Autodesk Inventor part; units mm, degrees
ref_plane "YZ Plane" through (0, 0, 0) normal (1, 0, 0) x (0, 1, 0)
ref_plane "XZ Plane" through (0, 0, 0) normal (0, 1, 0) x (-1, 0, 0)
ref_plane "XY Plane" through (0, 0, 0) normal (0, 0, 1) x (1, 0, 0)
sketch "Sketch1" plane through (0, 0, 0) normal (0, 0, 1) x (1, 0, 0)
  line L0 (3.25, -3.75) -> (-3.25, -3.75)
  line L1 (-3.75, -3.25) -> (-3.75, 3.25)
  line L2 (-3.25, 3.75) -> (3.25, 3.75)
  line L3 (3.75, 3.25) -> (3.75, -3.25)
  line L4 (3.75, -3.75) -> (-3.75, 3.75) construction
  line L5 (-3.75, -3.75) -> (3.75, 3.75) construction
  arc A0 (-3.25, 3.75) -> (-3.75, 3.25) centre (-3.25, 3.25) ccw
  arc A1 (-3.75, -3.25) -> (-3.25, -3.75) centre (-3.25, -3.25) ccw
  arc A2 (3.25, -3.75) -> (3.75, -3.25) centre (3.25, -3.25) ccw
  arc A3 (3.75, 3.25) -> (3.25, 3.75) centre (3.25, 3.25) ccw
  point P0 (0, 0)
  dimension "d0" = 7.5
  dimension "d1" = 0.5
extrude "Extrusion1" add sketch "Sketch1" along normal mid plane 3.02
sketch "Sketch2" plane through (0, 0, -1.51) normal (0, 0, -1) x (-1, 0, 0)
  line L0 (2.96, -3) -> (1.56, -3)
  line L1 (1.56, -3) -> (1.56, 3)
  line L2 (1.56, 3) -> (2.96, 3)
  line L3 (2.96, 3) -> (2.96, -3)
  line L4 (-1.56, -3) -> (-2.96, -3)
  line L5 (-2.96, -3) -> (-2.96, 3)
  line L6 (-2.96, 3) -> (-1.56, 3)
  line L7 (-1.56, 3) -> (-1.56, -3)
  line L8 (0, -3) -> (0, 3) construction
  point P0 (0, 0)
  point P1 (0, 0)
  dimension "d4" = 1.4
  dimension "d5" = 6
  dimension "d6" = 3.12
extrude "Extrusion2" add sketch "Sketch2" along normal blind 0.08
sketch "Sketch3" plane through (0, 0, 1.51) normal (0, 0, 1) x (1, 0, 0)
  line L0 (2.75, 2.5) -> (2.5, 2.5)
  line L1 (2.5, 2.5) -> (2.5, -2.5)
  line L2 (2.5, -2.5) -> (2.75, -2.5)
  line L3 (2.75, -2.5) -> (2.75, 2.5)
  line L4 (-2.5, 2.5) -> (-2.5, -2.5) construction
  spline S0 degree 4 poles (1.3361, 0.4296) (1.5722, 0.2536) (1.6111, 0.0081) (1.8752, -0.3041) (1.3349, -0.7643) (0.9016, -0.6061) (0.6086, -0.3512) (0.6279, 0.0301) (0.8528, 0.1857) (1.2221, 0.0137) (1.0663, -0.2096) (0.9971, -0.1716) (0.8339, -0.0827) (0.9372, -0.3475) (1.124, -0.4244) (1.5104, -0.4795) (1.4218, 0.1865) (0.9203, 0.4463) (0.2397, 0.5724) (-0.0703, -0.2361) (0.2655, -0.4716) (0.366, -0.6909) (0.4591, -0.7727) knots 0 0 0 0 0 0.123761 0.174234 0.226685 0.279962 0.33014 0.377129 0.419078 0.455262 0.487036 0.514913 0.545248 0.580512 0.622872 0.674906 0.733244 0.796807 0.860625 0.919671 1 1 1 1 1
  line L5 (0.3021, -0.6347) -> (0.6161, -0.9108) construction
  arc A0 (0.3672, -0.6474) -> (0.5952, -0.8479) centre (0.698, -0.5011) ccw construction
  spline S1 degree 4 poles (1.3361, 0.4296) (1.1748, 0.5523) (0.7861, 0.8379) (-0.1178, 0.7487) (-0.2762, -0.1647) (0.0057, -0.6403) (0.1538, -0.7727) knots 0 0 0 0 0 0.46045 0.670358 1 1 1 1 1
  line L6 (-0.0024, -0.6331) -> (0.3101, -0.9124) construction
  arc A1 (0.0518, -0.6477) -> (0.2895, -0.8602) centre (0.4983, -0.3874) ccw construction
  line L7 (0.4591, -0.7727) -> (0.1538, -0.7727)
  line L8 (1.4819, -0.2272) -> (1.2942, 0.2269) construction
  arc A2 (1.4343, -0.1846) -> (1.2905, 0.1631) centre (0.7871, -0.2485) ccw construction
  line L9 (-2.1499, 0.6983) -> (-2.1499, 0.9013)
  line L10 (-2.1499, 0.9013) -> (-2.5036, 0.9013)
  line L11 (-2.5036, 0.9013) -> (-2.5036, 1.2648)
  line L12 (-2.5036, 1.2648) -> (-2.1499, 1.2648)
  line L13 (-2.1499, 1.2648) -> (-2.1499, 1.9261)
  line L14 (-2.1499, 1.9261) -> (-1.8703, 1.9261)
  line L15 (-1.8703, 1.9261) -> (-1, 1.2769)
  line L16 (-1, 1.2769) -> (-1, 0.9013)
  line L17 (-1, 0.9013) -> (-1.8801, 0.9013)
  line L18 (-1.8801, 0.9013) -> (-1.8801, 0.6983)
  line L19 (-1.8801, 0.6983) -> (-2.1499, 0.6983)
  line L20 (-1.8801, 1.2648) -> (-1.3695, 1.2648)
  line L21 (-1.3695, 1.2648) -> (-1.8801, 1.6453)
  line L22 (-1.8801, 1.6453) -> (-1.8801, 1.2648)
  line L23 (-1.2978, -0.5646) -> (-2.5, 0.076)
  line L24 (-2.5, 0.076) -> (-2.5, 0.4941)
  line L25 (-2.5, 0.4941) -> (-1.2832, -0.1756)
  line L26 (-1.2832, -0.1756) -> (-1.2832, 0.5391)
  line L27 (-1.2832, 0.5391) -> (-1, 0.5391)
  line L28 (-1, 0.5391) -> (-1, -0.5646)
  line L29 (-1, -0.5646) -> (-1.2978, -0.5646)
  line L30 (-2.5, -1.9115) -> (-2.5, -0.809)
  line L31 (-2.5, -0.809) -> (-2.2557, -0.809)
  spline S2 degree 2 poles (-2.2557, -0.809) (-2.1438, -0.9487) (-1.9469, -1.1724) (-1.8582, -1.2563) knots 0 0 0 1 2 2 2
  spline S3 degree 2 poles (-1.8582, -1.2563) (-1.7427, -1.3669) (-1.5665, -1.4654) (-1.4741, -1.4654) knots 0 0 0 1 2 2 2
  spline S4 degree 2 poles (-1.4741, -1.4654) (-1.3695, -1.4654) (-1.2577, -1.3402) (-1.2577, -1.2283) knots 0 0 0 1 2 2 2
  spline S5 degree 2 poles (-1.2577, -1.2283) (-1.2577, -1.1712) (-1.2857, -1.0691) (-1.3075, -1.0168) knots 0 0 0 1 2 2 2
  spline S6 degree 2 poles (-1.3075, -1.0168) (-1.3306, -0.9658) (-1.3793, -0.8928) (-1.3914, -0.8746) knots 0 0 0 1 2 2 2
  line L32 (-1.3914, -0.8746) -> (-1.3914, -0.8454)
  line L33 (-1.3914, -0.8454) -> (-1.0644, -0.8454)
  spline S7 degree 2 poles (-1.0644, -0.8454) (-1.034, -0.9086) (-0.9708, -1.1785) (-0.9708, -1.3037) knots 0 0 0 1 2 2 2
  spline S8 degree 2 poles (-0.9708, -1.3037) (-0.9708, -1.5711) (-1.2091, -1.8458) (-1.4242, -1.8458) knots 0 0 0 1 2 2 2
  spline S9 degree 2 poles (-1.4242, -1.8458) (-1.5567, -1.8458) (-1.812, -1.7206) (-1.9579, -1.576) knots 0 0 0 1 2 2 2
  spline S10 degree 2 poles (-1.9579, -1.576) (-2.0478, -1.4848) (-2.1876, -1.3134) (-2.2168, -1.2757) knots 0 0 0 1 2 2 2
  line L34 (-2.2168, -1.2757) -> (-2.2168, -1.9115)
  line L35 (-2.2168, -1.9115) -> (-2.5, -1.9115)
  point P0 (0, 0)
  point P1 (-2.5, 0)
  point P2 (2.5, 0)
  point P3 (1.5897, 0.1222)
  point P4 (1.6836, -0.1324)
  point P5 (1.6666, -0.392)
  point P6 (1.348, -0.657)
  point P7 (0.9064, -0.5696)
  point P8 (0.6595, -0.2864)
  point P9 (0.6874, 0.0129)
  point P10 (0.9152, 0.1153)
  point P11 (1.131, -0.0524)
  point P12 (1.0559, -0.1747)
  point P13 (0.9784, -0.1613)
  point P14 (0.8944, -0.1391)
  point P15 (0.915, -0.2539)
  point P16 (1.1067, -0.4034)
  point P17 (1.3658, -0.3897)
  point P18 (1.3881, -0.0001)
  point P19 (0.911, 0.405)
  point P20 (0.2939, 0.3734)
  point P21 (0.0837, -0.1519)
  point P22 (0.2608, -0.5163)
  point P23 (1.0376, 0.6174)
  point P24 (0.5316, 0.7174)
  point P25 (0.0302, 0.4881)
  point P26 (-0.1564, -0.1329)
  dimension "d9" = 5
  dimension "d10" = 0.25
  dimension "d11" = 2.5
  dimension "d12" = 2.5
extrude "Extrusion3" add sketch "Sketch3" along normal blind 0.01
properties part number "Inductor_7575" material "Steel, Carbon"
Could you check a few things on this model? Use its own coordinates, in mm. Give positions to 0.01 mm unless a question says otherwise; leave off trailing zeros.
Q1. We'd pull the mould along X, two halves only. Please class faces 1 (the flat face through (0, 0, -1.51)), 2 (the flat face through (-2, 0, 1.52)), 3 (the flat face through (3.75, 0, 0)), 4 (the flat face through (0, 1, 1.51)): +X half, -X half, draft (parallel to the pull), parting line (faces both ways), or undercut.
Q2. If I drill on line 1 along Z through (x, y) = (-1.25, -3); line 2 along Z through (x, y) = (2, 2.75), over which ranges is the centre line in solid material (lowest first)?
Q3. I'm going to push a flat-ended pin straight in: P1, Ø1.5, axis at x = 0, y = 2, coming from the +Z side. Where does the tip first touch, or does it pass through?
Solution:
1. face 1: undercut
1. face 2: draft
1. face 3: +X half
1. face 4: undercut
2. line 1: z = -1.51 to 1.51
2. line 2: z = -1.59 to 1.51
3. P1: stops at z = 1.51
